Check sheet for the modelled part. Datum: model origin and axes. Units: mm. Face numbers are marked on the shaded views. Round coordinates to 2 decimals unless told otherwise and drop trailing zeros. Loops run counter-clockwise (first coordinate to the right, second up) from the corner with the lowest first, then second, coordinate; pieces in that order, holes last. Notation, with made-up numbers: (68.25, 43.25) - (77.25, 43.25) arc R26 ccw to (77.25, 61.25) - close; hole circle Ø6 at (72, -12). An arc over 180 degrees is marked (long way). Put each result on its own line as item: value.
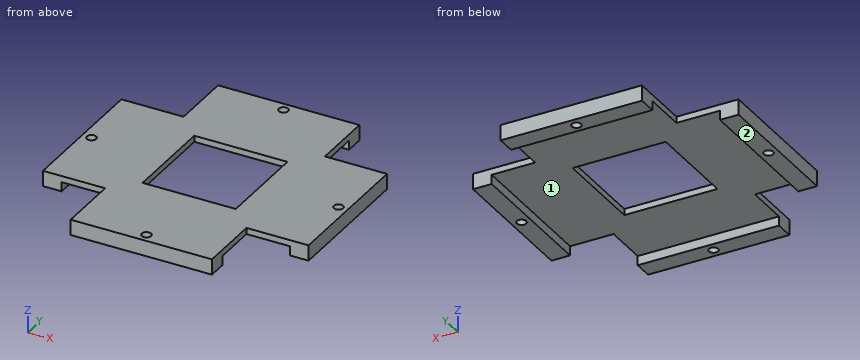
```python
from build123d import *

# Parameters (mm, degrees)
SKETCH033_W             = 30
SKETCH033_H             = 30
PAD009008_DEPTH         = 2
SKETCH034_W             = 45.5
SKETCH034_H             = 6
SKETCH034_W_2           = 6
SKETCH034_H_2           = 45.5
PAD009009_DEPTH         = 3
SKETCH035_R             = 1.5
POCKET003006_DEPTH      = 0.001
POCKET003006_DEPTH_BACK = 5.001


with BuildPart() as part:
    # Sketch033 → Pad009008 (new body)
    with BuildSketch(Plane(origin=(0, 0, 5), x_dir=(1, 0, 0), z_dir=(0, 0, -1))):
        Polygon((-22.75, 42.75), (22.75, 42.75), (22.75, 22.75), (42.75, 22.75), (42.75, -22.75), (22.75, -22.75), (22.75, -42.75), (-22.75, -42.75), (-22.75, -22.75), (-42.75, -22.75), (-42.75, 22.75), (-22.75, 22.75), align=None)
        Rectangle(SKETCH033_W, SKETCH033_H, mode=Mode.SUBTRACT)
    extrude(amount=PAD009008_DEPTH)

    # Sketch034 → Pad009009 (join)
    with BuildSketch(Plane(origin=(0, 0, 3), x_dir=(1, 0, 0), z_dir=(0, 0, -1))):
        with Locations((0, 39.75)):
            Rectangle(SKETCH034_W, SKETCH034_H)
        with Locations((0, -39.75)):
            Rectangle(SKETCH034_W, SKETCH034_H)
        with Locations((-39.75, 0)):
            Rectangle(SKETCH034_W_2, SKETCH034_H_2)
        with Locations((39.75, 0)):
            Rectangle(SKETCH034_W_2, SKETCH034_H_2)
    extrude(amount=PAD009009_DEPTH)

    # Sketch035 → Pocket003006 (cut, two sides)
    with BuildSketch(Plane.XY) as pocket003006_sk:
        with Locations((-39.75, 0)):
            Circle(SKETCH035_R)
        with Locations((0, 39.75)):
            Circle(SKETCH035_R)
        with Locations((39.75, 0)):
            Circle(SKETCH035_R)
        with Locations((0, -39.75)):
            Circle(SKETCH035_R)
    extrude(amount=-POCKET003006_DEPTH, mode=Mode.SUBTRACT)
    extrude(pocket003006_sk.sketch, amount=POCKET003006_DEPTH_BACK, mode=Mode.SUBTRACT)


solid = part.part
```
Item 1: Release check for a two-part mould opening along X. For the marked faces 1 and 2 record: +X half, -X half, draft (parallel to the pull), parting line (faces both ways), or undercut.
Filled sheet:
face 1: undercut
face 2: draft
Item 2: Thickness scan on line 1 (Y direction, x = 0, z = 2.8); line 2 (X direction, y = -20, z = 1.65). Record the ranges inside material, lowest first. Write a range as from..to.
Filled sheet:
line 1: -42.75..-41.25, -38.25..-36.75, 36.75..38.25, 41.25..42.75
line 2: -42.75..-36.75, 36.75..42.75
Item 3: Section check B-B on z = 2.1. Enter the section's corners in (x, y), then the cut area to 3 significant figures.
Filled sheet:
outline: (-42.75, -22.75) - (-36.75, -22.75) - (-36.75, 22.75) - (-42.75, 22.75) - close; (-22.75, -42.75) - (22.75, -42.75) - (22.75, -36.75) - (-22.75, -36.75) - close; (-22.75, 36.75) - (22.75, 36.75) - (22.75, 42.75) - (-22.75, 42.75) - close; (36.75, -22.75) - (42.75, -22.75) - (42.75, 22.75) - (36.75, 22.75) - close; hole circle Ø3 at (-39.75, 0); hole circle Ø3 at (0, -39.75); hole circle Ø3 at (0, 39.75); hole circle Ø3 at (39.75, 0)
area: 1,060 mm²
Item 4: Section check C-C on x = 6.5. Enter the section's corners in (y, z).
Filled sheet:
outline: (-42.75, 0) - (-36.75, 0) - (-36.75, 3) - (-15, 3) - (-15, 5) - (-42.75, 5) - close; (15, 3) - (36.75, 3) - (36.75, 0) - (42.75, 0) - (42.75, 5) - (15, 5) - close
Item 5: Go/stop test with flat-tipped pins: pin 1 (3 mm diameter, centred on x = 32.5, z = 4.5, fed in from +Y); pin 2 (4 mm diameter, centred on x = 0, y = 39.75, fed in from +Z). Record where each tip stops, or that it passes through.
Filled sheet:
pin 1: y = 22.75
pin 2: z = 5
Item 6: Section check A-A on y = 39.75. Enter the section's corners in (x, z).
Filled sheet:
outline: (-22.75, 0) - (-1.5, 0) - (-1.5, 5) - (-22.75, 5) - close; (1.5, 0) - (22.75, 0) - (22.75, 5) - (1.5, 5) - close
